from build123d import *
from build123d.topology import SkipClean

# Parameters (mm, degrees)
SKETCH1_R           = 100
BOSS_EXTRUDE2_DEPTH = 1120
SKETCH4_R           = 37.5
CUT_EXTRUDE1_DEPTH  = 1100
SKETCH6_R           = 30.030042901
CUT_EXTRUDE2_DEPTH  = 1129.893263334
SKETCH7_R           = 5
CUT_EXTRUDE3_DEPTH  = 1200
FILLET1_R           = 25
SKETCH8_W           = 276.180333513
SKETCH8_H           = 316.248560879
CUT_EXTRUDE4_DEPTH  = 65
SKETCH9_R           = 7.5
CUT_EXTRUDE5_DEPTH  = 2
BOSS_EXTRUDE3_START = 223.21458
BOSS_EXTRUDE3_DEPTH = 223.21458
SKETCH11_R          = 125
BOSS_EXTRUDE4_DEPTH = 10
SKETCH12_W          = 75
SKETCH12_H          = 228.21458
CUT_EXTRUDE6_DEPTH  = 123


with BuildPart() as part:
    # Sketch1 → Boss-Extrude2 (new body)
    with BuildSketch(Plane(origin=(0, 0, 0), x_dir=(1, 0, 0), z_dir=(0, 1, 0))):
        with Locations(Location((0, 0, 0), (0, 0, 270))):
            Circle(SKETCH1_R)
    extrude(amount=BOSS_EXTRUDE2_DEPTH)

    # Sketch4 → Cut-Extrude1 (cut)
    with BuildSketch(Plane(origin=(0, 1120, 0), x_dir=(1, 0, 0), z_dir=(0, 1, 0))):
        with Locations(Location((55, 0, 0), (0, 0, 270))):
            Circle(SKETCH4_R)
        with Locations(Location((0, 55, 0), (0, 0, 270))):
            Circle(SKETCH4_R)
        with Locations(Location((-55, 0, 0), (0, 0, 270))):
            Circle(SKETCH4_R)
        with Locations(Location((0, -55, 0), (0, 0, 270))):
            Circle(SKETCH4_R)
    extrude(amount=-CUT_EXTRUDE1_DEPTH, mode=Mode.SUBTRACT)

    # Sketch6 → Cut-Extrude2 (cut, through all)
    with BuildSketch(Plane(origin=(0, 1120, 0), x_dir=(1, 0, 0), z_dir=(0, 1, 0))):
        with Locations((-70.710678119, 70.710678119)):
            Circle(SKETCH6_R)
        with Locations((70.710678119, 70.710678119)):
            Circle(SKETCH6_R)
        with Locations((70.710678119, -70.710678119)):
            Circle(SKETCH6_R)
        with Locations((-70.710678119, -70.710678119)):
            Circle(SKETCH6_R)
    extrude(amount=-CUT_EXTRUDE2_DEPTH, mode=Mode.SUBTRACT)

    # Sketch7 → Cut-Extrude3 (cut)
    with BuildSketch(Plane(origin=(0, 1120, 0), x_dir=(1, 0, 0), z_dir=(0, 1, 0))):
        with Locations(Location((0, 0, 0), (0, 0, 270))):
            Circle(SKETCH7_R)
    extrude(amount=-CUT_EXTRUDE3_DEPTH, mode=Mode.SUBTRACT)

    # Fillet1
    fillet1_edges = [part.edges().sort_by_distance(p)[0] for p in [
        (-46.528605162, 560, 88.51603754),
        (-88.51603754, 560, 46.528605162),
        (88.51603754, 560, 46.528605162),
        (46.528605162, 560, 88.51603754),
        (46.528605162, 560, -88.51603754),
        (88.51603754, 560, -46.528605162),
        (-88.51603754, 560, -46.528605162),
        (-46.528605162, 560, -88.51603754),
    ]]
    fillet(fillet1_edges, radius=FILLET1_R)

    # Sketch8 → Cut-Extrude4 (cut)
    with BuildSketch(Plane(origin=(0, 1120, 0), x_dir=(1, 0, 0), z_dir=(0, 1, 0))):
        with Locations((9.785456368, -2.918303702)):
            Rectangle(SKETCH8_W, SKETCH8_H)
    extrude(amount=-CUT_EXTRUDE4_DEPTH, mode=Mode.SUBTRACT)

    # Sketch9 → Cut-Extrude5 (cut)
    with BuildSketch(Plane(origin=(0, 1055, 0), x_dir=(1, 0, 0), z_dir=(0, 1, 0))):
        with Locations(Location((0, 0, 0), (0, 0, 270))):
            Circle(SKETCH9_R)
    extrude(amount=-CUT_EXTRUDE5_DEPTH, mode=Mode.SUBTRACT)

    # Sketch10 → Boss-Extrude3 (add)
    with SkipClean():  # the faces are left unmerged after this step: merging them gives an invalid solid
        with BuildSketch(Plane.XZ.offset(BOSS_EXTRUDE3_START)):
            with BuildLine():
                ThreePointArc((20.990620884, 97.772152656), (0, 100), (-20.990620884, 97.772152656))
                ThreePointArc((-20.990620884, 97.772152656), (-35.556079582, 88.575114519), (-40.71464911, 72.139565913))
                ThreePointArc((-40.71464911, 72.139565913), (-49.476231144, 49.476231144), (-72.139565913, 40.71464911))
                ThreePointArc((-72.139565913, 40.71464911), (-88.575114519, 35.556079582), (-97.772152656, 20.990620884))
                ThreePointArc((-97.772152656, 20.990620884), (-100, 0), (-97.772152656, -20.990620884))
                ThreePointArc((-97.772152656, -20.990620884), (-88.575114519, -35.556079582), (-72.139565913, -40.71464911))
                ThreePointArc((-72.139565913, -40.71464911), (-49.476231144, -49.476231144), (-40.71464911, -72.139565913))
                ThreePointArc((-40.71464911, -72.139565913), (-35.556079582, -88.575114519), (-20.990620884, -97.772152656))
                ThreePointArc((-20.990620884, -97.772152656), (0, -100), (20.990620884, -97.772152656))
                ThreePointArc((20.990620884, -97.772152656), (35.556079582, -88.575114519), (40.71464911, -72.139565913))
                ThreePointArc((40.71464911, -72.139565913), (49.476231144, -49.476231144), (72.139565913, -40.71464911))
                ThreePointArc((72.139565913, -40.71464911), (88.575114519, -35.556079582), (97.772152656, -20.990620884))
                ThreePointArc((97.772152656, -20.990620884), (100, 0), (97.772152656, 20.990620884))
                ThreePointArc((97.772152656, 20.990620884), (88.575114519, 35.556079582), (72.139565913, 40.71464911))
                ThreePointArc((72.139565913, 40.71464911), (49.476231144, 49.476231144), (40.71464911, 72.139565913))
                ThreePointArc((40.71464911, 72.139565913), (35.556079582, 88.575114519), (20.990620884, 97.772152656))
            make_face()
        extrude(amount=-BOSS_EXTRUDE3_DEPTH)

    # Sketch11 → Boss-Extrude4 (add)
    with SkipClean():  # the faces are left unmerged after this step: merging them gives an invalid solid
        with BuildSketch(Plane.XZ.offset(223.21458)):
            with Locations(Location((0, 0, 0), (0, 0, 270))):
                Circle(SKETCH11_R)
        extrude(amount=-BOSS_EXTRUDE4_DEPTH)

    # Sketch12 → Cut-Extrude6 (cut, symmetric)
    with SkipClean():  # the faces are left unmerged after this step: merging them gives an invalid solid
        with BuildSketch(Plane(origin=(0, 0, 0), x_dir=(0, 0, -1), z_dir=(1, 0, 0))):
            with Locations((0, -99.10729)):
                Rectangle(SKETCH12_W, SKETCH12_H)
        extrude(amount=CUT_EXTRUDE6_DEPTH, both=True, mode=Mode.SUBTRACT)


solid = part.part
Verification items for the finished model (mm, model axes). A direction names the side the tool comes from. Round coordinates to 2 decimals unless told otherwise and drop trailing zeros. Loops run counter-clockwise (first coordinate to the right, second up) from the corner with the lowest first, then second, coordinate; pieces in that order, holes last. Notation, with made-up numbers: (15, 40.5) - (37, 40.5) arc R7 cw to (37, 49.5) - close; hole circle Ø8 at (77, -37.75). An arc over 180 degrees is marked (long way). Answer in a Markdown table with one row per item. Add a question column.
Q1. Section check C-C on z = 55. Enter the section's corners in (x, y).
Q2. Section check B-B on y = -36. Enter the section's corners in (x, z), plus the area to 3 significant figures.
Q3. Section check A-A on x = 55. Enter the section's corners in (y, z).
Q4. Section check D-D on y = 810. State how many separate pieces and enclosed holes the cut face has, plus the area to 3 significant figures.
Q5. Release check for a two-part mould opening along X. For faces 5 (the face through (100, 528, 0)), 6 (the face through (1, 15, -8)), 7 (the face through (-54, 20, -1)) record: pulls with the +X half, pulls with the -X half, needs draft (parallel to the pull), parting line crosses it, or undercut.
Q6. Tool access check on faces 1 (the face through (1, 20, 54)), 2 (the face through (2, -223.215, 2)), 3 (the face through (-100, 528, 0)), 4 (the face through (1, -101, 37.5)). Record the directions out of +Z, -Z, +X, -X, +Y, -Y that give a thin tool (end or side, any length) a straight path to the whole face; none if there is none.
Q7. Material ranges on line 1 (X direction, y = 344, z = 0); line 2 (Y direction, x = 44, z = -5); line 3 (X direction, y = 953, z = -33.5), recorded low to high.
Q8. Gauge pin test, flat ends, axial feed: pin 1 (7.5 mm diameter, centred on x = -2, z = 1.5, fed in from +Y); pin 2 (22.5 mm diameter, centred on x = 15, z = 46.5, fed in from +Y); pin 3 (8 mm diameter, centred on y = 235, z = -10.5, fed in from -X). Record the tip position at first contact, or that the pin passes through.
Found:
| question | item | result |
|---|---|---|
| 1 | outline | (-112.25, -223.21) - (112.25, -223.21) - (112.25, -213.21) - (45.12, -213.21) - (45.12, 1055) - (37.5, 1055) - (37.5, 20) - (-37.5, 20) - (-37.5, 1055) - (-45.12, 1055) - (-45.12, -213.21) - (-112.25, -213.21) - close |
| 2 | outline | (-85.64, -37.5) arc R25 ccw to (-72.14, -40.71) arc R30.03 cw to (-40.71, -72.14) arc R25 ccw to (-20.99, -97.77) arc R100 ccw to (20.99, -97.77) arc R25 ccw to (40.71, -72.14) arc R30.03 cw to (72.14, -40.71) arc R25 ccw to (85.64, -37.5) - close; (-85.64, 37.5) - (85.64, 37.5) arc R25 ccw to (72.14, 40.71) arc R30.03 cw to (40.71, 72.14) arc R25 ccw to (20.99, 97.77) arc R100 ccw to (-20.99, 97.77) arc R25 ccw to (-40.71, 72.14) arc R30.03 cw to (-72.14, 40.71) arc R25 ccw to start |
| 2 | area | 10,700 mm² |
| 3 | outline | (-223.21, -112.25) - (-213.21, -112.25) - (-213.21, -45.12) - (1055, -45.12) - (1055, -37.5) - (20, -37.5) - (20, 37.5) - (1055, 37.5) - (1055, 45.12) - (-213.21, 45.12) - (-213.21, 112.25) - (-223.21, 112.25) - close; hole (-213.21, -37.5) - (15, -37.5) - (15, 37.5) - (-213.21, 37.5) - close |
| 4 | separate pieces | 1 |
| 4 | enclosed holes | 5 |
| 4 | area | 7,510 mm² |
| 5 | face 5 | pulls with the +X half |
| 5 | face 6 | needs draft |
| 5 | face 7 | undercut |
| 6 | face 1 | +Y |
| 6 | face 2 | +Z, -Z, +X, -X, -Y |
| 6 | face 3 | -X, +Y |
| 6 | face 4 | +X, -X |
| 7 | line 1 | x = -100 to -92.5, -17.5 to -5, 5 to 17.5, 92.5 to 100 |
| 7 | line 2 | y = -223.21 to -213.21, 15 to 20 |
| 7 | line 3 | x = -90.93 to -71.85, -38.15 to -30.72, 30.72 to 38.15, 71.85 to 90.93 |
| 8 | pin 1 | stops at y = 1053 |
| 8 | pin 2 | stops at y = 20 |
| 8 | pin 3 | stops at x = -99.79 |
